Here's how the part is built. I have some questions about the finished solid (model axes, mm). A direction names the side the tool comes from. Round coordinates to 2 decimals unless told otherwise and drop trailing zeros. Order: outer loops, then holes, each group sorted by start corner. A loop starts at its lowest first (then second) coordinate and runs counter-clockwise, first axis right, second up. Notation, with made-up numbers: M 27.5,-36.5 L 82.5,-36.5 A25 cw 82.5,-21.5 Z; hole C 9,-22.75 d10. An arc over 180 degrees is marked long. Write item = value, one per line. Start each with the question number.
Item 1: I want a section at B-B, the plane y = 5.75. List the corners of the cut face in (x, z) for me (3 decimals), plus the area to 3 significant figures.
Item 2: We'd pull the mould along X, two halves only. Please class faces 4 (the face through (12, -0.755, 0)), 5 (the face through (0.11, 8.117, -26.248)): pulls with the +X half, pulls with the -X half, needs draft (parallel to the pull), parting line crosses it, or undercut.
Item 3: I want a section at A-A, the plane z = 0. List the corners of the cut face in (x, y) for me (3 decimals), plus the area to 3 significant figures.
Item 4: I want a section at D-D, the plane y = 13. List the corners of the cut face in (x, z) for me (3 decimals).
Item 5: For faces 1 (the face through (8, 10.245, 5)), 2 (the face through (12, 16.745, 0)), 3 (the face through (8, 2.245, -5)), which set-ups out of +Z, -Z, +X, -X, +Y, -Y let a thin tool reach every point of the face, with its end or its side?
Item 6: I'm going to push flat-ended pins straight in: P1, Ø2, axis at y = 13.5, z = 3.5, coming from the +X side; P2, Ø12, axis at x = -22.5, z = 19.5, coming from the +Y side (3 decimals); P3, Ø10, axis at x = -8, y = 3.5, coming from the +Z side; P4, Ø8, axis at y = 8.5, z = 21, coming from the -X side. Where does each tip first touch, or does it pass through?
Item 7: Please list where these lines run through material, in increasing order: L1, parallel to Z at x = 20.5, y = 13; L2, parallel to Z at x = 21.5, y = 11.25; L3, parallel to Z at x = -1.5, y = 6.5.
Item 8: I want a section at C-C, the plane x = 0. State how many separate pieces and enclosed holes the cut face has, plus the area to 3 significant figures.
```python
from build123d import *

# Parameters (mm, degrees)
SKETCH_3_R          = 2.5
CUT_EXTRUDE_1_DEPTH = 17.5
CHAMFER_1_SIZE      = 0.2


with BuildPart() as part:
    # ｽｹｯﾁ2 → 回転1 (revolve)
    with BuildSketch(Plane.XY, mode=Mode.PRIVATE) as revolve_1_sk:
        Polygon((-9.075, 10.244997288), (-9.075, 2.244997288), (-11, 2.244997288), (-11, -0.755002712), (-28.5, -0.755002712), (-28.5, 16.744997288), (-11, 16.744997288), (-11, 10.244997288), align=None)
    revolve(revolve_1_sk.sketch.rotate(Axis((0, 0, 0), (0, 1, 0)), 270), axis=Axis((0, 0, 0), (0, 1, 0)))

    # ｽｹｯﾁ3 → ｶｯﾄ - 押し出し1 (cut)
    with BuildSketch(Plane(origin=(0, 16.744997288, 0), x_dir=(1, 0, 0), z_dir=(0, 1, 0))):
        with Locations(Location((0, 23.75, 0), (0, 0, 270))):
            Circle(SKETCH_3_R)
        with Locations(Location((20.56810334, 11.875, 0), (0, 0, 270))):
            Circle(SKETCH_3_R)
        with Locations(Location((20.56810334, -11.875, 0), (0, 0, 270))):
            Circle(SKETCH_3_R)
        with Locations(Location((0, -23.75, 0), (0, 0, 270))):
            Circle(SKETCH_3_R)
        with Locations(Location((-20.56810334, -11.875, 0), (0, 0, 270))):
            Circle(SKETCH_3_R)
        with Locations(Location((-20.56810334, 11.875, 0), (0, 0, 270))):
            Circle(SKETCH_3_R)
    extrude(amount=-CUT_EXTRUDE_1_DEPTH, mode=Mode.SUBTRACT)

    # 面取り1
    chamfer_1_edges = [part.edges().sort_by_distance(p)[0] for p in [
        (0, 16.744997288, 11),
        (0, 16.744997288, 28.5),
        (0, -0.755002712, 28.5),
        (0, -0.755002712, 11),
        (0, 2.244997288, 9.075),
        (0, 10.244997288, 9.075),
    ]]
    chamfer(chamfer_1_edges, length=CHAMFER_1_SIZE)


solid = part.part
```
Filled in:
q1.outline = C 0,0 d57; hole C -20.568,-11.875 d5; hole C -20.568,11.875 d5; hole C 0,0 d18.15; hole C 0,-23.75 d5; hole C 0,23.75 d5; hole C 20.568,-11.875 d5; hole C 20.568,11.875 d5
q1.area = 2,180 mm^2
q2.face_4 = needs draft
q2.face_5 = undercut
q3.outline = M -28.5,-0.555 L -28.3,-0.755 L -11.2,-0.755 L -11,-0.555 L -11,2.245 L -9.275,2.245 L -9.075,2.445 L -9.075,10.045 L -9.275,10.245 L -11,10.245 L -11,16.545 L -11.2,16.745 L -28.3,16.745 L -28.5,16.545 Z; M 9.075,2.445 L 9.275,2.245 L 11,2.245 L 11,-0.555 L 11.2,-0.755 L 28.3,-0.755 L 28.5,-0.555 L 28.5,16.545 L 28.3,16.745 L 11.2,16.745 L 11,16.545 L 11,10.245 L 9.275,10.245 L 9.075,10.045 Z
q3.area = 643 mm^2
q4.outline = C 0,0 d57; hole C -20.568,-11.875 d5; hole C -20.568,11.875 d5; hole C 0,0 d22; hole C 0,-23.75 d5; hole C 0,23.75 d5; hole C 20.568,-11.875 d5; hole C 20.568,11.875 d5
q5.face_1 = +Y
q5.face_2 = +Z, -Z, +X, -X, +Y
q5.face_3 = -Y
q6.P1 = 28.39
q6.P2 = 16.745
q6.P3 = 28.34
q6.P4 = -22.87
q7.L1 = -19.8 to -14.37, -9.38 to 9.38, 14.37 to 19.8
q7.L2 = -18.71 to -14.19, -9.56 to 9.56, 14.19 to 18.71
q7.L3 = -28.46 to -25.75, -21.75 to -8.95, 8.95 to 21.75, 25.75 to 28.46
q8.separate_pieces = 4
q8.enclosed_holes = 0
q8.area = 468 mm^2
